from build123d import *

# Parameters (mm, degrees)
SKETCH1_W                = 250
SKETCH1_H                = 60
BOSS_EXTRUDE1_DEPTH      = 20
BOSS_EXTRUDE3_DEPTH      = 17.5
BOSS_EXTRUDE3_DEPTH_BACK = 17.5
SKETCH4_R                = 40
BOSS_EXTRUDE5_DEPTH      = 80
BOSS_EXTRUDE5_DRAFT      = -23
SKETCH4_4_R              = 15
CUT_EXTRUDE3_DEPTH       = 168


with BuildPart() as part:
    # Sketch1 → Boss-Extrude1 (new body)
    with BuildSketch(Plane(origin=(0, 0, 0), x_dir=(1, 0, 0), z_dir=(0, 1, 0))):
        Rectangle(SKETCH1_W, SKETCH1_H)
    extrude(amount=BOSS_EXTRUDE1_DEPTH)

    # Sketch3 → Boss-Extrude3 (add, two sides: drawn at the far end of the back side and taken through both)
    with BuildSketch(Plane.XY.offset(-BOSS_EXTRUDE3_DEPTH_BACK)):
        with BuildLine():
            Line((105, 20), (-45, 20))
            Line((-45, 20), (40.410284884, 338.755522675))
            add(Edge.make_bspline(
                [(40.410284884, 338.755522675), (80, 370), (105, 370)],
                knots=[0, 0, 0, 1, 1, 1], degree=2))
            Line((105, 370), (105, 20))
        make_face()
    extrude(amount=BOSS_EXTRUDE3_DEPTH + BOSS_EXTRUDE3_DEPTH_BACK)


with BuildPart() as boss_extrude5_tool:
    # Sketch4 → Boss-Extrude5 (with draft: the straight prism first)
    with BuildSketch(Plane(origin=(105, 0, 0), x_dir=(0, 0, -1), z_dir=(1, 0, 0))):
        with Locations((0, 320)):
            Circle(SKETCH4_R)
    extrude(amount=-BOSS_EXTRUDE5_DEPTH)
    # Boss-Extrude5: the draft: its side faces are tilted about the plane it starts from
    boss_extrude5_sides = [boss_extrude5_tool.faces().sort_by_distance(p)[0] for p in [
        (65, 320, 40),
    ]]
    draft(boss_extrude5_sides, Plane(origin=(105, 0, 0), x_dir=(0, 0, -1), z_dir=(1, 0, 0)), BOSS_EXTRUDE5_DRAFT)


with BuildPart() as part_1:
    add(part.part)

    # Boss-Extrude5: add boss_extrude5_tool
    add(boss_extrude5_tool.part)

    # Sketch4_4 → Cut-Extrude3 (cut)
    with BuildSketch(Plane(origin=(105, 0, 0), x_dir=(0, 0, -1), z_dir=(1, 0, 0))):
        with Locations(Location((0, 320, 0), (0, 0, 90))):
            Circle(SKETCH4_4_R)
    extrude(amount=-CUT_EXTRUDE3_DEPTH, mode=Mode.SUBTRACT)


solid = part_1.part
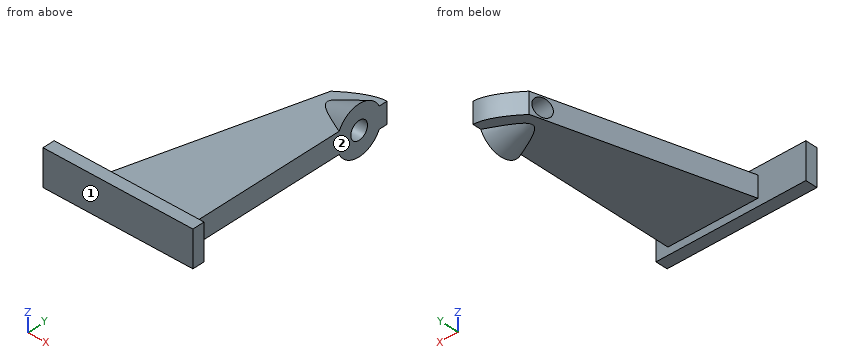
The listing builds one solid part. Answer for the finished solid, in the listing's coordinates (mm). Face numbers are marked on the shaded views. A direction names the side the tool comes from. Round coordinates to 2 decimals unless told otherwise and drop trailing zeros. Order: outer loops, then holes, each group sorted by start corner. A loop starts at its lowest first (then second) coordinate and runs counter-clockwise, first axis right, second up. Notation, with made-up numbers: (-26, 3.25) -> (-13, 3.25) arc R24 cw to (-13, 21.25) -> close; hole circle Ø10 at (45, -2). An arc over 180 degrees is marked (long way). Put each result on its own line as item: value.
Q1. Consider line 1 along Z through (x, y) = (48, 320); line 2 along X through (y, z) = (337, 0); line 3 along Y through (x, z) = (-22, -25). Determine where each line is inside the solid, lowest interval first.
Results list:
line 1: -17.5 to -15, 15 to 17.5
line 2: 39.94 to 105
line 3: 0 to 20
Q2. Each of these flat-tipped pins is pushed along its axis until it touches: P1, Ø18, axis at x = 36, z = 3.5, coming from the +Y side; P2, Ø3, axis at x = -60.5, z = -5.5, coming from the +Y side; P3, Ø6, axis at x = 17.5, y = 7, coming from the -Z side. Where does it stop, or does it pass through?
Results list:
P1: y = 342.31
P2: y = 20
P3: z = -30
Q3. Section A-A, the plane y = 320 is taken. Write down the section's boundary in (x, z).
Results list:
outline: (35.38, -17.5) -> (51.99, -17.5) -> (105, -40) -> (105, -15) -> (35.38, -15) -> close; (35.38, 15) -> (105, 15) -> (105, 40) -> (51.99, 17.5) -> (35.38, 17.5) -> close
Q4. Section C-C, the plane y = 73 is taken. Write down the section's boundary in (x, z), and give its area (3 significant figures).
Results list:
outline: (-30.8, -17.5) -> (105, -17.5) -> (105, 17.5) -> (-30.8, 17.5) -> close
area: 4,750 mm^2
Q5. Section B-B, the plane x = -93.5 is taken. Write down the section's boundary in (y, z).
Results list:
outline: (0, -30) -> (20, -30) -> (20, 30) -> (0, 30) -> close
Q6. Section D-D, the plane x = -7.5 is taken. Write down the section's boundary in (y, z), and give its area (3 significant figures).
Results list:
outline: (0, -30) -> (20, -30) -> (20, -17.5) -> (159.95, -17.5) -> (159.95, 17.5) -> (20, 17.5) -> (20, 30) -> (0, 30) -> close
area: 6,100 mm^2
Q7. Which of the six approach directions +Z, -Z, +X, -X, +Y, -Y give full straight-line access (tool end or side, diameter ignored) to the marked faces 1 and 2?
Results list:
face 1: +Z, -Z, +X, -X, -Y
face 2: +Z, -Z, +X, +Y
